from build123d import *

# Parameters (mm, degrees)
SKETCH1_R               = 5.08
BOSS_EXTRUDE1_DEPTH     = 12.7
SKETCH2_R               = 2.999994
CUT_EXTRUDE1_DEPTH      = 9.541256
SKETCH3_R               = 3.175
BOSS_EXTRUDE2_DEPTH     = 12.065
CUT_EXTRUDE2_DEPTH      = 7.62
CUT_EXTRUDE2_DEPTH_BACK = 7.62
SKETCH4_R               = 0.79375
SKETCH7_W               = 0.79375
SKETCH7_H               = 4.200130206
CUT_EXTRUDE3_DEPTH      = 12.065


with BuildPart() as part:
    # Sketch1 → Boss-Extrude1 (new body)
    with BuildSketch(Plane.YZ):
        with Locations(Location((0, 0, 0), (0, 0, 270))):
            Circle(SKETCH1_R)
    extrude(amount=BOSS_EXTRUDE1_DEPTH)

    # Sketch2 → Cut-Extrude1 (cut)
    with BuildSketch(Plane.YZ.offset(12.7)):
        with Locations(Location((0, 0, 0), (0, 0, 270))):
            Circle(SKETCH2_R)
    extrude(amount=-CUT_EXTRUDE1_DEPTH, mode=Mode.SUBTRACT)

    # Sketch3 → Boss-Extrude2 (add)
    with BuildSketch(Plane(origin=(0, 0, 0), x_dir=(0, -1, 0), z_dir=(-1, 0, 0))):
        with Locations(Location((0, 0, 0), (0, 0, 270))):
            Circle(SKETCH3_R)
    extrude(amount=BOSS_EXTRUDE2_DEPTH)

    # Sketch4 → Cut-Extrude2 (cut, two sides: drawn at the far end of the back side and taken through both)
    with BuildSketch(Plane(origin=(0, 0, 0), x_dir=(0, 1, 0), z_dir=(0, 0, 1)).offset(-CUT_EXTRUDE2_DEPTH_BACK)):
        with Locations(Location((0, -6.35, 0), (0, 0, 90))):
            Circle(SKETCH4_R)
    extrude(amount=CUT_EXTRUDE2_DEPTH + CUT_EXTRUDE2_DEPTH_BACK, mode=Mode.SUBTRACT)

    # Sketch7 → Cut-Extrude3 (cut)
    with BuildSketch(Plane(origin=(-12.065, 0, 0), x_dir=(0, -1, 0), z_dir=(-1, 0, 0))):
        with Locations((-2.778125, 0)):
            Rectangle(SKETCH7_W, SKETCH7_H)
    extrude(amount=-CUT_EXTRUDE3_DEPTH, mode=Mode.SUBTRACT)


solid = part.part
Could you check a few things on this model? Use its own coordinates, in mm. A direction names the side the tool comes from. Give positions to 0.01 mm unless a question says otherwise; leave off trailing zeros. Order: outer loops, then holes, each group sorted by start corner. A loop starts at its lowest first (then second) coordinate and runs counter-clockwise, first axis right, second up.
Item 1: For faces 4 (the face through (8, 0.9, -2.86)), 5 (the face through (0, -1.1, -3.3)), 6 (the face through (5.593, -0.238, 3.971)), which set-ups out of +Z, -Z, +X, -X, +Y, -Y let a thin tool reach every point of the face, with its end or its side?
Item 2: I'm going to push flat-ended pins straight in: pin 1 (1 mm diameter, centred on x = -5, y = 1, fed in from -Z); pin 2 (4 mm diameter, centred on x = -1.5, z = -3.5, fed in from +Y); pin 3 (2 mm diameter, centred on x = -7.5, z = -0.5, fed in from +Y). Where does each tip first touch, or does it pass through?
Item 3: If we section it at B-B, the plane x = 6.35: Write out the boundary of the cut face in (y, z).
Item 4: If we section it at C-C, the plane z = 0: Write out the boundary of the cut face in (x, y) (3 decimals), plus the area to 3 significant figures.
Item 5: If we mould it in two halves opening along Z, with no side actions, what happens to faces 1 (the face through (3.159, 0, 0)), 2 (the face through (-6, 2.381, 0)), 3 (the face through (-5.948, -3.173, -0.107))? For each: pulls with the +Z half, pulls with the -Z half, needs draft (parallel to the pull), parting line crosses it, or undercut.
Item 6: If we section it at A-A, the plane y = 0: Write out the boundary of the cut face in (x, z) (3 decimals).
Item 7: I need wall thicknesses on line 1 (Y direction, x = 5.5, z = 0); line 2 (X direction, y = 0, z = -4.1). Which ranges of each line are inside material? Lowest first, please.
Item 8: If we section it at D-D, the plane y = -2: Write out the boundary of the cut face in (x, z) (3 decimals).
Values:
1. face 4: +X
1. face 5: -X
1. face 6: +Z, -Z
2. pin 1: stops at z = -3.14
2. pin 2: stops at y = 4.59
2. pin 3: stops at y = 2.38
3. outline: (-0.79, -5.02) - (-0.79, -2.89) arc R3 cw to (-0.79, 2.89) - (-0.79, 5.02) arc R5.08 ccw to start; (0.79, -5.02) arc R5.08 ccw to (0.79, 5.02) - (0.79, 2.89) arc R3 cw to (0.79, -2.89) - close
4. outline: (-12.065, -3.175) - (0, -3.175) - (0, -5.08) - (12.7, -5.08) - (12.7, -3) - (3.159, -3) - (3.159, 3) - (12.7, 3) - (12.7, 5.08) - (0, 5.08) - (0, 2.381) - (-12.065, 2.381) - close
4. area: 139 mm2
5. face 1: undercut
5. face 2: needs draft
5. face 3: parting line crosses it
6. outline: (-12.065, -3.175) - (0, -3.175) - (0, -5.08) - (5.556, -5.08) - (5.556, -3) - (3.159, -3) - (3.159, 3) - (5.556, 3) - (5.556, 5.08) - (0, 5.08) - (0, 3.175) - (-12.065, 3.175) - close; (7.144, -5.08) - (12.7, -5.08) - (12.7, -3) - (7.144, -3) - close; (7.144, 3) - (12.7, 3) - (12.7, 5.08) - (7.144, 5.08) - close
7. line 1: y = -5.08 to -3, 3 to 5.08
7. line 2: x = 0 to 5.56, 7.14 to 12.7
8. outline: (-12.065, -2.466) - (0, -2.466) - (0, -4.67) - (12.7, -4.67) - (12.7, -2.236) - (3.159, -2.236) - (3.159, 2.236) - (12.7, 2.236) - (12.7, 4.67) - (0, 4.67) - (0, 2.466) - (-12.065, 2.466) - close
